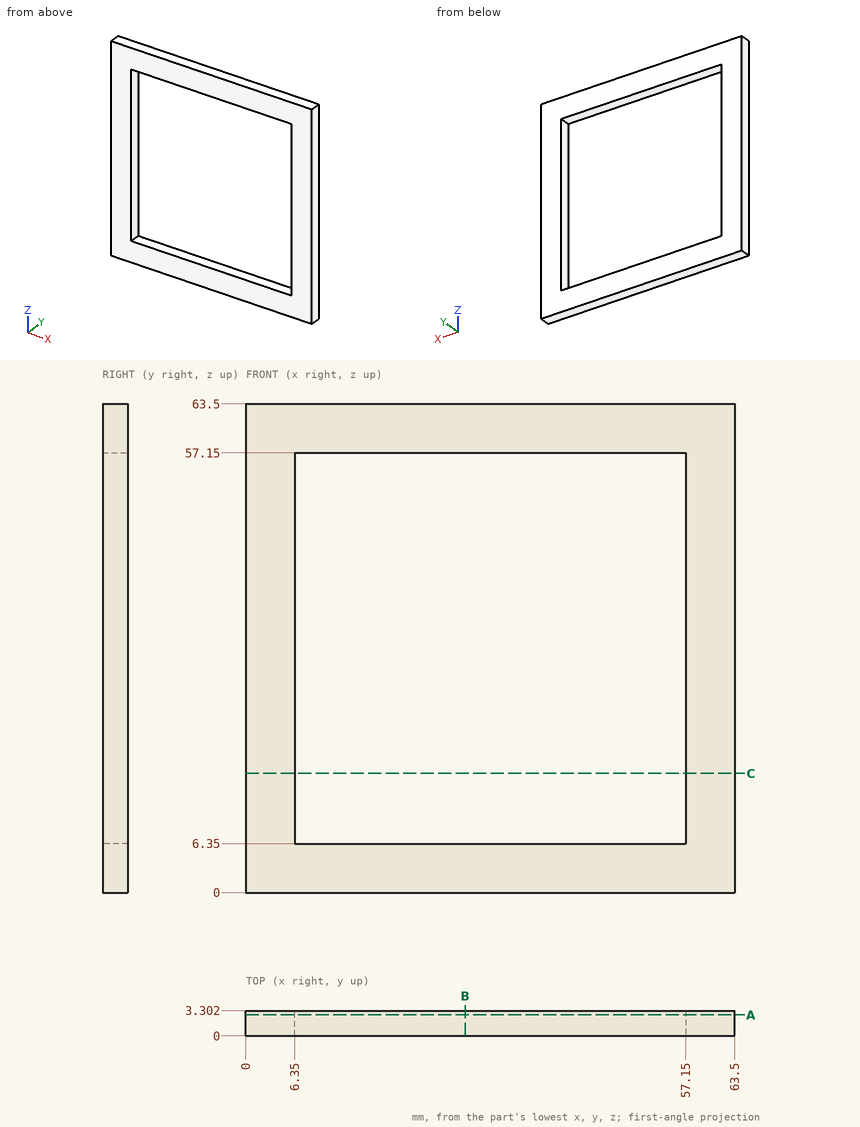
For this review, use the dimensioned drawing (mm, ordinates from the lowest corner) and the shaded views. Give positions to 0.01 mm unless a question says otherwise; leave off trailing zeros. Order: outer loops, then holes, each group sorted by start corner. A loop starts at its lowest first (then second) coordinate and runs counter-clockwise, first axis right, second up. Notation, with made-up numbers: (-7, 37) - (-2, 37) arc R34 cw to (-2, 67) - close; hole circle Ø2 at (-27.75, -39). An arc over 180 degrees is marked (long way). Use a Markdown table: item, result. Add a question column.
(1) Clearance check with a flat-ended pin moving along its axis: P1, Ø1.7, axis at y = 2.5, z = 28, coming from the -X side. State where the tip first meets the part, or that it passes through.
(2) Add section B-B on x = 28.5. Give the boundary of the cut face in (y, z).
(3) Add section C-C on z = 15.5. Give the boundary of the cut face in (x, y), then the cut area to 3 significant figures.
(4) Wall thickness on probe 1 along Z at (x, y) = (30, 2.9): over which ranges is the line inside the solid? List them lowest first. Write a range as [from, to].
(5) Add section A-A on y = 2.75. Give the boundary of the cut face in (x, z), then the cut area to 3 significant figures.
Report:
| question | item | result |
|---|---|---|
| 1 | P1 | stops at x = 0 |
| 2 | outline | (0, 0) - (3.3, 0) - (3.3, 6.35) - (0, 6.35) - close; (0, 57.15) - (3.3, 57.15) - (3.3, 63.5) - (0, 63.5) - close |
| 3 | outline | (0, 0) - (6.35, 0) - (6.35, 3.3) - (0, 3.3) - close; (57.15, 0) - (63.5, 0) - (63.5, 3.3) - (57.15, 3.3) - close |
| 3 | area | 41.9 mm² |
| 4 | probe 1 | z = [0, 6.35], [57.15, 63.5] |
| 5 | outline | (0, 0) - (63.5, 0) - (63.5, 63.5) - (0, 63.5) - close; hole (6.35, 6.35) - (57.15, 6.35) - (57.15, 57.15) - (6.35, 57.15) - close |
| 5 | area | 1,450 mm² |
